For this review, take the finished solid that the model builds, in its own axes (mm). A direction names the side the tool comes from. Round coordinates to 2 decimals unless told otherwise and drop trailing zeros. Order: outer loops, then holes, each group sorted by start corner. A loop starts at its lowest first (then second) coordinate and runs counter-clockwise, first axis right, second up. Notation, with made-up numbers: M -39,-2.5 L -30,-2.5 A18 ccw -30,29.5 Z; hole C -18.75,-4.75 d3. An arc over 180 degrees is marked long. Write item = value, one per line. Start each with the question number.
from build123d import *

# Parameters (mm, degrees)
CROQUIS1_R              = 3
SALIENTE_EXTRUIR1_DEPTH = 3
REDONDEO1_R             = 2
REDONDEO2_R             = 2


with BuildPart() as part:
    # Croquis1 → Saliente-Extruir1 (new body)
    with BuildSketch(Plane(origin=(0, 0, 0), x_dir=(1, 0, 0), z_dir=(0, 1, 0))):
        with BuildLine():
            Line((59.968853779, -6.466358732), (82.968853779, -6.466358732))
            ThreePointArc((82.968853779, -6.466358732), (93.968853779, 4.533641268), (82.968853779, 15.533641268))
            Line((82.968853779, 15.533641268), (67.968853779, 15.533641268))
            ThreePointArc((67.968853779, 15.533641268), (16.376491879, 36.535254234), (-19.031146221, -6.466358732))
            Line((-19.031146221, -6.466358732), (-13.031146221, -6.466358732))
            ThreePointArc((-13.031146221, -6.466358732), (23.468853779, 18.795009604), (59.968853779, -6.466358732))
        make_face()
        with Locations(Location((82.968853779, 4.533641268, 0), (0, 0, 270))):
            Circle(CROQUIS1_R, mode=Mode.SUBTRACT)
    extrude(amount=SALIENTE_EXTRUIR1_DEPTH)

    # Redondeo1
    redondeo1_edges = [part.edges().sort_by_distance(p)[0] for p in [
        (59.968853779, 1.5, 6.466358732),
    ]]
    fillet(redondeo1_edges, radius=REDONDEO1_R)

    # Redondeo2
    redondeo2_edges = [part.edges().sort_by_distance(p)[0] for p in [
        (-13.031146221, 1.5, 6.466358732),
    ]]
    fillet(redondeo2_edges, radius=REDONDEO2_R)


solid = part.part
(1) We need section D-D, the plane x = 21. Write out the cut boundary in (y, z), then the cut area to 3 significant figures.
(2) We need section B-B, the plane z = -12.5. Write out the cut boundary in (x, y), then the cut area to 3 significant figures.
(3) Draft analysis for pull direction X (two halves, no side actions). For faces 4 (the cylindrical face through (17.187, 1.479, -36.733)), 5 (the cylindrical face through (-13.266, 1.521, 6.121)), 6 (the flat face through (-17, 1, 6.466)), state which applies: released by +X, released by -X, zero draft, split by the parting line, or undercut.
(4) We need section C-C, the plane z = -6. Write out the cut boundary in (x, y).
(5) We need section A-A, the plane y = 0.7. Write out the cut boundary in (x, z) (3 decimals).
(6) For line 1 along X through (y, z) = (2.45, -3); line 2 along X through (y, z) = (1.9, 0); line 3 along X through (y, z) = (0.7, -11), list the stretches that pass through material, from the lowest coordinate up.
(7) For faces 1 (the cylindrical face through (60.23, 1.52, 6.14)), 2 (the flat face through (76, 1, -15.534)), 3 (the cylindrical face through (85.943, 1.479, -4.924)), list the 3-axis set-ups (+Z, -Z, +X, -X, +Y, -Y) from which the entire face can be reached by the end or side of a thin tool; tool diameter is ignored.
Values:
q1.outline = M 0,-37.46 L 3,-37.46 L 3,-18.72 L 0,-18.72 Z
q1.area = 56.2 mm²
q2.outline = M -13.88,0 L 2.22,0 L 2.22,3 L -13.88,3 Z; M 44.71,0 L 90.55,0 L 90.55,3 L 44.71,3 Z
q2.area = 186 mm²
q3.face_4 = split by the parting line
q3.face_5 = undercut
q3.face_6 = zero draft
q4.outline = M -16.63,0 L -5.42,0 L -5.42,3 L -16.63,3 Z; M 52.35,0 L 80.35,0 L 80.35,3 L 52.35,3 Z; M 85.59,0 L 93.87,0 L 93.87,3 L 85.59,3 Z
q5.outline = M -19.031,6.466 A47 ccw 67.969,-15.534 L 82.969,-15.534 A11 ccw 82.969,6.466 L 61.328,6.466 A2 ccw 59.481,5.234 A39 cw -12.543,5.234 A2 ccw -14.39,6.466 Z; hole C 82.969,-4.534 d6
q6.line_1 = -17.54 to -7.88, 54.81 to 80.39, 85.55 to 93.86
q6.line_2 = -18.23 to -9.89, 56.83 to 92.99
q6.line_3 = -14.62 to 0.08, 46.86 to 91.87
q7.face_1 = +Z, +Y, -Y
q7.face_2 = -Z, +X, +Y, -Y
q7.face_3 = +Y, -Y
